Can you work these out from the model? Positions are in its coordinate system, mm. Face numbers are marked on the shaded views. A direction names the side the tool comes from. Give positions to 0.01 mm unless a question says otherwise; leave off trailing zeros. Order: outer loops, then holes, each group sorted by start corner. A loop starts at its lowest first (then second) coordinate and runs counter-clockwise, first axis right, second up. Notation, with made-up numbers: (33.5, 34) - (71.5, 34) arc R28 cw to (71.5, 68) - close; hole circle Ø5 at (51, 62.5). An arc over 180 degrees is marked (long way). Use one line per item in the form item = value. Start each with the question number.
1) Suppose I cut it at A-A, the plane z = 0.5. Write out the boundary of the cut face in (x, y).
2) We'd pull the mould along X, two halves only. Please class the marked faces 1 and 2: released by +X, released by -X, zero draft, split by the parting line, or undercut.
3) For pin 1 (4 mm diameter, centred on x = -7, y = -4.5, fed in from +Z); pin 2 (1 mm diameter, centred on y = 8, z = -2.5, fed in from -X); pin 3 (4 mm diameter, centred on x = -11, z = 0.5, fed in from -Y); pin 4 (4 mm diameter, centred on x = -4.5, z = 3, fed in from +Y) (3 decimals), each with a flat end and sliding along its axis, tell me the tip position at first contact or that it passes through.
4) Please list where these lines run through material, in increasing order: probe 1 along Y at (x, z) = (0, -3.45); probe 2 along Z at (x, y) = (5.5, -7.5); probe 3 along Z at (x, y) = (7.5, -0.25).
5) Which directions (+Z, -Z, +X, -X, +Y, -Y) give clear straight access to the entire face, cutting with the end or side of a thin tool? Please do the marked faces 3 and 4.
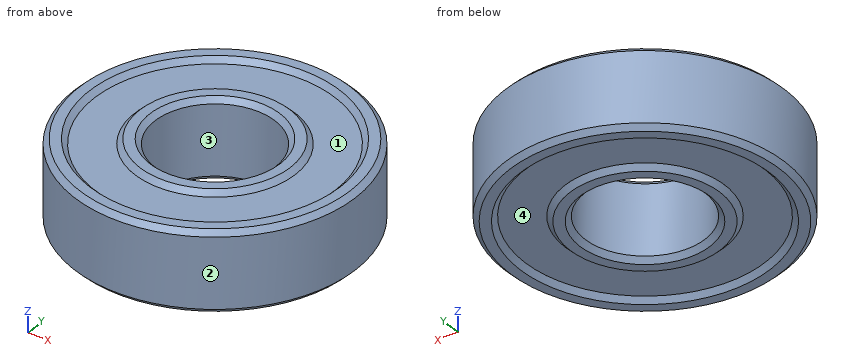
```python
from build123d import *

# Parameters (mm, degrees)
SKETCH1_R           = 14
SKETCH1_R_2         = 6
BOSS_EXTRUDE1_DEPTH = 4
CUT_EXTRUDE1_START  = -4
SKETCH1_3_R         = 12
SKETCH1_3_R_2       = 8
CUT_EXTRUDE1_DEPTH  = 0.5
CUT_EXTRUDE2_START  = 3.5
SKETCH1_4_R         = 12
SKETCH1_4_R_2       = 8
CUT_EXTRUDE2_DEPTH  = 0.5
CHAMFER1_SIZE       = 0.5


with BuildPart() as part:
    # Sketch1 → Boss-Extrude1 (new, symmetric)
    with BuildSketch(Plane.XY):
        Circle(SKETCH1_R)
        Circle(SKETCH1_R_2, mode=Mode.SUBTRACT)
    extrude(amount=BOSS_EXTRUDE1_DEPTH, both=True)

    # Sketch1<3> → Cut-Extrude1 (cut)
    with BuildSketch(Plane.XY.offset(CUT_EXTRUDE1_START)):
        Circle(SKETCH1_3_R)
        Circle(SKETCH1_3_R_2, mode=Mode.SUBTRACT)
    extrude(amount=CUT_EXTRUDE1_DEPTH, mode=Mode.SUBTRACT)

    # Sketch1<4> → Cut-Extrude2 (cut)
    with BuildSketch(Plane.XY.offset(CUT_EXTRUDE2_START)):
        Circle(SKETCH1_4_R)
        Circle(SKETCH1_4_R_2, mode=Mode.SUBTRACT)
    extrude(amount=CUT_EXTRUDE2_DEPTH, mode=Mode.SUBTRACT)

    # Chamfer1
    chamfer1_edges = [part.edges().sort_by_distance(p)[0] for p in [
        (-8, 0, -4),
        (-12, 0, -4),
        (-14, 0, -4),
        (-12, 0, 4),
        (-8, 0, 4),
        (-14, 0, 4),
        (-6, 0, -4),
        (-6, 0, 4),
    ]]
    chamfer(chamfer1_edges, length=CHAMFER1_SIZE - 0.0001)  # a hair under: the kernel refuses the full size


solid = part.part
```
Result sheet:
q1.outline = circle Ø28 at (0, 0); hole circle Ø12 at (0, 0)
q2.face_1 = undercut
q2.face_2 = split by the parting line
q3.pin_1 = 4
q3.pin_2 = -11.82
q3.pin_3 = -10.72
q3.pin_4 = 13.775
q4.probe_1 = -14 to -6, 6 to 14
q4.probe_2 = -3.5 to 3.5
q4.probe_3 = -4 to 4
q5.face_3 = +Z, -Z
q5.face_4 = -Z
